Could you check a few things on this model? Use its own coordinates, in mm. A direction names the side the tool comes from. Round coordinates to 2 decimals unless told otherwise and drop trailing zeros. Write each loop counter-clockwise with the first axis right and the second up, starting at its lowest first coordinate (ties: lowest second). Pieces come first, ordered by that corner, then holes. Notation, with made-up numbers: (-14, 28.25) -> (23, 28.25) arc R26 cw to (23, 50.25) -> close; hole circle Ø2 at (-32, 51). An arc over 180 degrees is marked (long way). Return JSON: item names as keys, results as strings.
from build123d import *

# Parameters (mm, degrees)
F0_W     = 76.2
F0_H     = 95.25
F1_DEPTH = 796.925
F2_W     = 95.25
F2_H     = 95.25
F3_DEPTH = 38.1
F4_W     = 76.2
F4_H     = 47.625
F5_DEPTH = 76.201
F6_W     = 95.25
F6_H     = 95.25
F7_DEPTH = 38.1


with BuildPart() as f1:
    # F0 (on Front) → F1 (new body)
    with BuildSketch(Plane.XZ):
        with Locations((38.1, 47.625)):
            Rectangle(F0_W, F0_H)
    extrude(amount=F1_DEPTH)

    # F2 (on face) → F3 (cut)
    with BuildSketch(Plane.YZ.offset(76.2)):
        with Locations((-749.3, 47.625)):
            Rectangle(F2_W, F2_H)
    extrude(amount=-F3_DEPTH, mode=Mode.SUBTRACT)

    # F4 (on face) → F5 (cut, through all)
    with BuildSketch(Plane.YZ.offset(76.2)):
        with Locations((-425.45, 71.4375)):
            Rectangle(F4_W, F4_H)
        with Locations((-38.1, 71.4375)):
            Rectangle(F4_W, F4_H)
    extrude(amount=-F5_DEPTH, mode=Mode.SUBTRACT)

    # F6 (on face) → F7 (cut)
    with BuildSketch(Plane.YZ.offset(76.2)):
        with Locations((-168.275, 47.625)):
            Rectangle(F6_W, F6_H)
    extrude(amount=-F7_DEPTH, mode=Mode.SUBTRACT)


solid = f1.part
1) I want a section at C-C, the plane x = 17. Please give me the cut outline in (y, z) (3 decimals), and give its area (3 significant figures).
Return value:
{"outline": "(-796.925, 0) -> (0, 0) -> (0, 47.625) -> (-76.2, 47.625) -> (-76.2, 95.25) -> (-387.35, 95.25) -> (-387.35, 47.625) -> (-463.55, 47.625) -> (-463.55, 95.25) -> (-796.925, 95.25) -> close", "area": "68,600 mm²"}
2) If I drill on probe 1 along Y at (x, z) = (41, 61.5) (3 decimals); probe 2 along Y at (x, z) = (5, 48) (3 decimals); probe 3 along Y at (x, z) = (57.5, 47.5) (3 decimals), over which ranges is the centre line in solid material (lowest first)? Write a range as [from, to].
Return value:
{"probe 1": "[-701.675, -463.55], [-387.35, -215.9], [-120.65, -76.2]", "probe 2": "[-796.925, -463.55], [-387.35, -76.2]", "probe 3": "[-701.675, -215.9], [-120.65, 0]"}
3) I want a section at D-D, the plane z = 24. Please give me the cut outline in (x, y) (3 decimals).
Return value:
{"outline": "(0, -796.925) -> (38.1, -796.925) -> (38.1, -701.675) -> (76.2, -701.675) -> (76.2, -215.9) -> (38.1, -215.9) -> (38.1, -120.65) -> (76.2, -120.65) -> (76.2, 0) -> (0, 0) -> close"}
4) I want a section at B-B, the plane z = 76.5. Please give me the cut outline in (x, y) (3 decimals).
Return value:
{"outline": "(0, -796.925) -> (38.1, -796.925) -> (38.1, -701.675) -> (76.2, -701.675) -> (76.2, -463.55) -> (0, -463.55) -> close; (0, -387.35) -> (76.2, -387.35) -> (76.2, -215.9) -> (38.1, -215.9) -> (38.1, -120.65) -> (76.2, -120.65) -> (76.2, -76.2) -> (0, -76.2) -> close"}
5) I want a section at A-A, the plane x = 46.5. Please give me the cut outline in (y, z) (3 decimals).
Return value:
{"outline": "(-701.675, 0) -> (-215.9, 0) -> (-215.9, 95.25) -> (-387.35, 95.25) -> (-387.35, 47.625) -> (-463.55, 47.625) -> (-463.55, 95.25) -> (-701.675, 95.25) -> close; (-120.65, 0) -> (0, 0) -> (0, 47.625) -> (-76.2, 47.625) -> (-76.2, 95.25) -> (-120.65, 95.25) -> close"}
6) For faces 1 (the face through (39, -426, 47.625)), 2 (the face through (38.1, -750, 48)), 3 (the face through (39, -39, 47.625)), 4 (the face through (38.1, -169, 48)), which set-ups out of +Z, -Z, +X, -X, +Y, -Y let a thin tool reach every point of the face, with its end or its side?
Return value:
{"face 1": "+Z, +X, -X", "face 2": "+Z, -Z, +X, -Y", "face 3": "+Z, +X, -X, +Y", "face 4": "+Z, -Z, +X"}
7) Will these pins go through, and if not, where does the flat tip stop? pin 1 Ø19 at (x, z) = (58.5, 29.5) entering from -Y (3 decimals); pin 2 Ø14.5 at (x, z) = (43, 81) entering from +Y.
Return value:
{"pin 1": "y = -701.675", "pin 2": "y = -76.2"}
